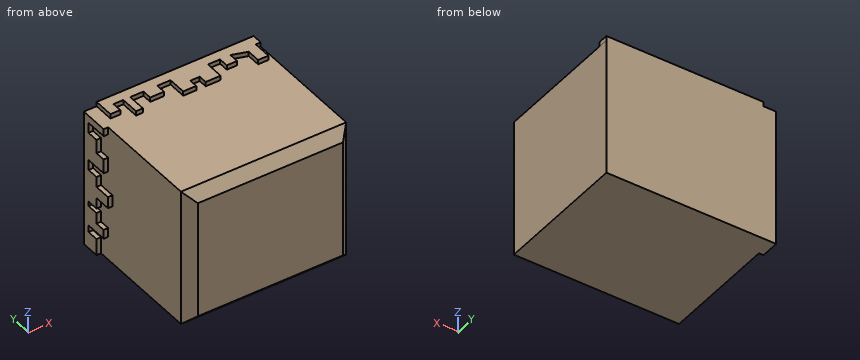
```python
from build123d import *

# Parameters (mm, degrees)
F0_W     = 83.653443
F0_H     = 73.160328
F1_DEPTH = 69.596
F3_DEPTH = 2.286
F5_DEPTH = 2.286
F6_SIZE  = 5.08


with BuildPart() as f1:
    # F0 (on Top) → F1 (new body)
    with BuildSketch(Plane.XY):
        with Locations((-2.769016, 10.784589)):
            Rectangle(F0_W, F0_H)
    extrude(amount=F1_DEPTH)

    # F2 (on face) → F3 (join)
    with BuildSketch(Plane(origin=(-44.595737, 0, 0), x_dir=(0, -1, 0), z_dir=(-1, 0, 0))):
        Polygon((-47.364753, 0), (-38.037542, 0), (-38.037542, 8.452787), (-43.867048, 8.452787), (-43.867048, 11.950491), (-32.790981, 11.950491), (-32.790981, 16.6141), (-38.037542, 16.6141), (-38.037542, 22.152131), (-43.867048, 22.152131), (-43.867048, 24.483934), (-38.037542, 24.483934), (-38.037542, 30.021966), (-29.584754, 30.021966), (-29.584754, 35.851479), (-38.037542, 35.851479), (-38.037542, 41.098036), (-43.867048, 41.098036), (-43.867048, 46.344589), (-32.790981, 46.344589), (-32.790981, 53.631473), (-38.037542, 53.631473), (-38.037542, 60.626887), (-43.867048, 60.626887), (-43.867048, 65.873444), (-32.790981, 65.873444), (-32.790981, 69.596), (-47.364753, 69.596), align=None)
    extrude(amount=F3_DEPTH)

    # F4 (on face) → F5 (join)
    with BuildSketch(Plane.XY.offset(69.596)):
        Polygon((39.057706, 47.364753), (-40.410984, 47.364753), (-40.410984, 37.163116), (-35.455901, 37.163116), (-35.455901, 42.118195), (-30.50082, 42.118195), (-30.50082, 32.790981), (-27.003115, 32.790981), (-27.003115, 42.118195), (-20.299181, 42.118195), (-20.299181, 37.163116), (-13.303772, 37.163116), (-13.303772, 42.118195), (-6.599837, 42.118195), (-6.599837, 32.790981), (0, 32.790981), (0, 37.163116), (4.767703, 37.163116), (4.767703, 32.790981), (12.346066, 32.790981), (12.346066, 42.118195), (18.467048, 42.118195), (18.467048, 37.163116), (23.713607, 37.163116), (23.713607, 42.118195), (31.291965, 39.640656), (31.291965, 32.790981), (36.538523, 32.790981), (36.538523, 42.118195), (39.057706, 42.118195), align=None)
    extrude(amount=F5_DEPTH)

    # F6
    f6_edges = [f1.edges().sort_by_distance(p)[0] for p in [
        (-2.769016, -25.795575, 69.596),
        (-44.595737, -25.795575, 34.798),
        (-2.769016, -25.795575, 0),
        (39.057706, -25.795575, 34.798),
    ]]
    chamfer(f6_edges, length=F6_SIZE)


solid = f1.part
```
The model under review builds one solid part; all positions refer to its coordinate system, in mm. Coordinates: 2 decimals unless noted, no trailing zeros. Write each loop counter-clockwise with the first axis right and the second up, starting at its lowest first coordinate (ties: lowest second). Pieces come first, ordered by that corner, then holes. Notation, with made-up numbers: (57, 72) -> (96, 72) arc R26 cw to (96, 111) -> close; hole circle Ø5 at (44.5, 73). An arc over 180 degrees is marked (long way). One line per item, written item: value. Start each with the question number.
Q1. To check wall thickness, follow probe 1 along Z at (x, y) = (-8, 31); probe 2 along X at (y, z) = (6.5, 52); probe 3 along Y at (x, z) = (0, 4). State the ranges of each line that lie inside material, in increasing order.
Q2. Clearance check with flat-ended pins moving along their axes: P1, Ø8, axis at y = 4, z = 64.5, coming from the -X side; P2, Ø2, axis at x = 27.5, y = 24, coming from the +Z side; P3, Ø2.5, axis at x = -46.5, z = 51, coming from the -Y side; P4, Ø1.1, axis at x = -46, y = 40, coming from the -Z side. State where each tip first meets the part, or that it passes through.
Q3. Add section B-B, the plane z = 10. Give the boundary of the cut face in (x, y), then the cut area to 3 significant figures.
Q4. Add section C-C, the plane y = 19. Give the boundary of the cut face in (x, z), then the cut area to 3 significant figures.
Q5. Add section A-A, the plane x = 15. Give the boundary of the cut face in (y, z), then the cut area to 3 significant figures.
Response:
1. probe 1: 0 to 69.6
1. probe 2: -44.6 to 39.06
1. probe 3: -24.72 to 47.36
2. P1: x = -44.6
2. P2: z = 69.6
2. P3: y = 32.79
2. P4: z = 0
3. outline: (-46.88, 43.87) -> (-44.6, 43.87) -> (-44.6, -20.72) -> (-39.52, -25.8) -> (33.98, -25.8) -> (39.06, -20.72) -> (39.06, 47.36) -> (-46.88, 47.36) -> close
3. area: 6,100 mm²
4. outline: (-44.6, 0) -> (39.06, 0) -> (39.06, 69.6) -> (-44.6, 69.6) -> close
4. area: 5,820 mm²
5. outline: (-25.8, 5.08) -> (-20.72, 0) -> (47.36, 0) -> (47.36, 71.88) -> (42.12, 71.88) -> (42.12, 69.6) -> (-20.72, 69.6) -> (-25.8, 64.52) -> close
5. area: 5,080 mm²
